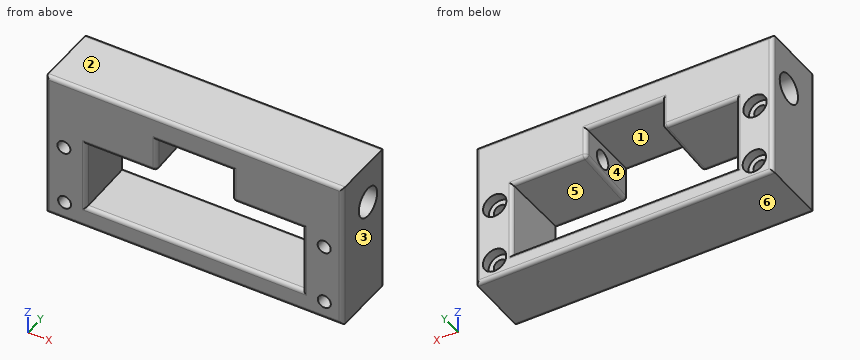
from build123d import *

# Parameters (mm, degrees)
SKETCH_1_W              = 80
SKETCH_1_H              = 40
EXTRUDE_1_DEPTH         = 18
CUT_EXTRUDE_1_DEPTH     = 49.207883173
DRAFT_1_ANGLE           = -3.5
HOLE_WIZARD_3_5_3_5_1_D = 3.5
M8X1_0_1_D              = 5
M8X1_0_1_DEPTH          = 29.8
M8X1_0_1_CBORE_D        = 8
M8X1_0_1_CBORE_DEPTH    = 22
M8X1_0_2_D              = 5
M8X1_0_2_DEPTH          = 80
M8X1_0_2_CBORE_D        = 8
M8X1_0_2_CBORE_DEPTH    = 22
FILLET_1_R              = 1
SKETCH_9_R              = 3.15
CUT_EXTRUDE_2_DEPTH     = 2.5


with BuildPart() as part:
    # ｽｹｯﾁ1 → ﾎﾞｽ - 押し出し1 (new body)
    with BuildSketch(Plane(origin=(0, 18, 0), x_dir=(1, 0, 0), z_dir=(0, 1, 0))):
        Rectangle(SKETCH_1_W, SKETCH_1_H)
    extrude(amount=-EXTRUDE_1_DEPTH)

    # ｽｹｯﾁ2 → ｶｯﾄ - 押し出し1 (cut, through all)
    with BuildSketch(Plane.XZ):
        Polygon((-10.2, 13.2), (-10.2, 4.099072837), (-29.099072837, 4.099072837), (-29.099072837, -14.099072837), (29.099072837, -14.099072837), (29.099072837, 4.099072837), (10.2, 4.099072837), (10.2, 13.2), align=None)
    extrude(amount=-CUT_EXTRUDE_1_DEPTH, mode=Mode.SUBTRACT)

    # 抜き勾配1
    draft_1_faces = [part.faces().sort_by_distance(p)[0] for p in [
        (-19.649536419, 9, 4.099072837),
        (-29.099072837, 9, -5),
        (0, 9, -14.099072837),
        (29.099072837, 9, -5),
        (19.649536419, 9, 4.099072837),
    ]]
    draft(draft_1_faces, Plane(origin=(0, 0, 0), x_dir=(0, 0, -1), z_dir=(0, -1, 0)), DRAFT_1_ANGLE)

    # Ø3.5 (3.5) 直径の穴1 (through all)
    with Locations(Plane(origin=(0, 18, 0), x_dir=(1, 0, 0), z_dir=(0, 1, 0))):
        with Locations((-35.186293991, -1), (-35, 15), (34.958159373, -1), (35, 15)):
            Hole(HOLE_WIZARD_3_5_3_5_1_D / 2)

    # M8x1.0 ねじ穴1
    with Locations(Plane(origin=(40, 0, 0), x_dir=(0, 0, -1), z_dir=(1, 0, 0))):
        with Locations((-8.8, 11)):
            CounterBoreHole(M8X1_0_1_D / 2, M8X1_0_1_CBORE_D / 2, M8X1_0_1_CBORE_DEPTH, depth=M8X1_0_1_DEPTH)

    # M8x1.0 ねじ穴2
    with Locations(Plane.ZY.offset(40)):
        with Locations((8.8, 11)):
            CounterBoreHole(M8X1_0_2_D / 2, M8X1_0_2_CBORE_D / 2, M8X1_0_2_CBORE_DEPTH, depth=M8X1_0_2_DEPTH)

    # ﾌｨﾚｯﾄ1
    fillet_1_edges = [part.edges().sort_by_distance(p)[0] for p in [
        (40, 0, 0),
        (0, 0, -20),
        (0, 18, 13.2),
        (10.2, 18, 9.2),
        (20.2, 18, 5.2),
        (10.2, 9, 4.649536419),
        (30.2, 18, -5),
        (0, 18, -15.2),
        (-30.2, 18, -5),
        (-20.2, 18, 5.2),
        (-10.2, 18, 9.2),
        (-10.2, 9, 4.649536419),
        (0, 0, 13.2),
        (-10.2, 0, 8.649536419),
        (-19.649536419, 0, 4.099072837),
        (-29.099072837, 0, -5),
        (0, 0, -14.099072837),
        (29.099072837, 0, -5),
        (19.649536419, 0, 4.099072837),
        (10.2, 0, 8.649536419),
        (-40, 0, 0),
        (0, 18, -20),
        (40, 18, 0),
        (0, 18, 20),
        (-40, 18, 0),
        (0, 0, 20),
    ]]
    fillet(fillet_1_edges, radius=FILLET_1_R)

    # ｽｹｯﾁ9 → ｶｯﾄ - 押し出し2 (cut)
    with BuildSketch(Plane(origin=(0, 18, 0), x_dir=(1, 0, 0), z_dir=(0, 1, 0))):
        with Locations(Location((35, 15, 0), (0, 0, 270))):
            Circle(SKETCH_9_R)
        with Locations(Location((34.958159373, -1, 0), (0, 0, 270))):
            Circle(SKETCH_9_R)
        with Locations(Location((-35, 15, 0), (0, 0, 270))):
            Circle(SKETCH_9_R)
        with Locations(Location((-35.186293991, -1, 0), (0, 0, 270))):
            Circle(SKETCH_9_R)
    extrude(amount=-CUT_EXTRUDE_2_DEPTH, mode=Mode.SUBTRACT)


solid = part.part
For this review, take the finished solid that the model builds, in its own axes (mm). Face numbers are marked on the shaded views. A direction names the side the tool comes from. Round coordinates to 2 decimals unless told otherwise and drop trailing zeros. Write each loop counter-clockwise with the first axis right and the second up, starting at its lowest first coordinate (ties: lowest second). Pieces come first, ordered by that corner, then holes. Notation, with made-up numbers: (-3, 48) - (40, 48) arc R24 ccw to (40, 63) - close; hole circle Ø11 at (-26, 75). An arc over 180 degrees is marked (long way). Use a Markdown table: item, result.
Q1. We need section A-A (x = -21). Give the boundary of the cut face in (y, z).
Derived:
| item | result |
|---|---|
| outline | (0, -19) arc R1 ccw to (1, -20) - (17, -20) arc R1 ccw to (18, -19) - (18, -16.14) arc R1 ccw to (17.06, -15.14) - (1.06, -14.16) arc R1 ccw to (0, -15.16) - close; (0, 5.16) arc R1 ccw to (1.06, 4.16) - (17.06, 5.14) arc R1 ccw to (18, 6.14) - (18, 19) arc R1 ccw to (17, 20) - (1, 20) arc R1 ccw to (0, 19) - close; hole circle Ø8 at (11, 8.8) |
Q2. We need section D-D (z = -11). Give the boundary of the cut face in (x, y), plus the area to 3 significant figures.
Derived:
| item | result |
|---|---|
| outline | (-40, 1) arc R1 ccw to (-39, 0) - (-30.16, 0) arc R1 ccw to (-29.16, 1.06) - (-30.14, 17.06) arc R1 ccw to (-31.14, 18) - (-39, 18) arc R1 ccw to (-40, 17) - close; (29.16, 1.06) arc R1 ccw to (30.16, 0) - (39, 0) arc R1 ccw to (40, 1) - (40, 17) arc R1 ccw to (39, 18) - (31.14, 18) arc R1 ccw to (30.14, 17.06) - close |
| area | 371 mm2 |
Q3. We need section B-B (z = 8.8). State how many separate pieces and enclosed holes the cut face has, plus the area to 3 significant figures.
Derived:
| item | result |
|---|---|
| separate pieces | 4 |
| enclosed holes | 0 |
| area | 641 mm2 |
Q4. Wall thickness on line 1 along X through (y, z) = (5, -15); line 2 along X through (y, z) = (1.25, -6); line 3 along Z through (x, y) = (35, 4.75): over which ranges is each line inside the solid? List them lowest first.
Derived:
| item | result |
|---|---|
| line 1 | x = -40 to -36.75, -33.25 to 33.25, 36.75 to 40 |
| line 2 | x = -40 to -29.18, 29.18 to 40 |
| line 3 | z = -20 to -16.75, -13.25 to -0.75, 2.75 to 20 |
Q5. We need section C-C (x = 7). Give the boundary of the cut face in (y, z).
Derived:
| item | result |
|---|---|
| outline | (0, -19) arc R1 ccw to (1, -20) - (17, -20) arc R1 ccw to (18, -19) - (18, -16.14) arc R1 ccw to (17.06, -15.14) - (1.06, -14.16) arc R1 ccw to (0, -15.16) - close; (0, 14.2) arc R1 ccw to (1, 13.2) - (17, 13.2) arc R1 ccw to (18, 14.2) - (18, 19) arc R1 ccw to (17, 20) - (1, 20) arc R1 ccw to (0, 19) - close |
Q6. The part is to be moulded in two halves that separate along Z. For the marked faces 1, 2 and 3, say which applies: pulls with the +Z half, pulls with the -Z half, needs draft (parallel to the pull), parting line crosses it, or undercut.
Derived:
| item | result |
|---|---|
| face 1 | undercut |
| face 2 | pulls with the +Z half |
| face 3 | needs draft |
Q7. Machinability: for the marked faces 4, 5 and 6, which of the approach directions +Z, -Z, +X, -X, +Y, -Y give a long, thin tool a straight path to every point of the face, cutting with its end or side? Answer none if there is none.
Derived:
| item | result |
|---|---|
| face 4 | +Y, -Y |
| face 5 | +Y |
| face 6 | -Z, +X, -X, +Y, -Y |
Q8. Clearance check with flat-ended pins moving along their axes: pin 1 (4 mm diameter, centred on y = 11, z = 9.5, fed in from -X); pin 2 (5.5 mm diameter, centred on x = -35, z = -15, fed in from +Y); pin 3 (6 mm diameter, centred on y = 10.5, z = 9, fed in from +X). State where each tip first meets the part, or that it passes through.
Derived:
| item | result |
|---|---|
| pin 1 | stops at x = -18 |
| pin 2 | stops at y = 15.5 |
| pin 3 | stops at x = 18 |
